```python
from build123d import *

# Parameters (mm, degrees)
EXTRUDE_6_DEPTH = 60


with BuildPart() as part:
    # Эскиз1 → Повернуть7 (revolve)
    with BuildSketch(Plane.XY, mode=Mode.PRIVATE) as revolve_7_sk:
        Polygon((120, 0), (0, 0), (0, -100), (90, -100), (90, -355), (20, -355), (20, -400), (40, -400), (115.131397208, -379.868602792), (120, -375), align=None)
    revolve(revolve_7_sk.sketch.rotate(Axis((0, 0, 0), (1, 0, 0)), 270), axis=Axis((0, 0, 0), (1, 0, 0)))

    # Эскиз3 → Бобышка-Вытянуть6 (add)
    with BuildSketch(Plane.ZY.offset(-90)):
        with BuildLine():
            ThreePointArc((-48.745403909, -87.314864701), (-70.710678119, -70.710678119), (-87.314864701, -48.745403909))
            ThreePointArc((-87.314864701, -48.745403909), (-86.141576096, -54.996690721), (-88.975283359, -60.691012112))
            Line((-88.975283359, -60.691012112), (-257.169911814, -228.885640567))
            ThreePointArc((-257.169911814, -228.885640567), (-264.676174548, -231.805098536), (-271.900138456, -228.243980661))
            ThreePointArc((-271.900138456, -228.243980661), (-226.413585645, -273.42620254), (-173.542276552, -309.690294083))
            ThreePointArc((-173.542276552, -309.690294083), (-203.646432227, -265.561170399), (-186.637594429, -214.921865676))
            Line((-186.637594429, -214.921865676), (-60.691012112, -88.975283359))
            ThreePointArc((-60.691012112, -88.975283359), (-54.996690721, -86.141576096), (-48.745403909, -87.314864701))
        make_face()
        with BuildLine():
            ThreePointArc((-96.209138584, -27.272727273), (-100, 0), (-96.209138584, 27.272727273))
            ThreePointArc((-96.209138584, 27.272727273), (-99.799825551, 22.022759648), (-105.830052443, 20))
            Line((-105.830052443, 20), (-343.693177122, 20))
            ThreePointArc((-343.693177122, 20), (-351.065274929, 23.243360753), (-353.655298198, 30.869565217))
            ThreePointArc((-353.655298198, 30.869565217), (-353.440103732, -33.242940208), (-341.697027586, -96.271186441))
            ThreePointArc((-341.697027586, -96.271186441), (-331.779877601, -43.780331217), (-283.94541729, -20))
            Line((-283.94541729, -20), (-105.830052443, -20))
            ThreePointArc((-105.830052443, -20), (-99.799825551, -22.022759648), (-96.209138584, -27.272727273))
        make_face()
        with BuildLine():
            ThreePointArc((-87.314864701, 48.745403909), (-70.710678119, 70.710678119), (-48.745403909, 87.314864701))
            ThreePointArc((-48.745403909, 87.314864701), (-54.996690721, 86.141576096), (-60.691012112, 88.975283359))
            Line((-60.691012112, 88.975283359), (-228.885640567, 257.169911814))
            ThreePointArc((-228.885640567, 257.169911814), (-231.805098536, 264.676174548), (-228.243980661, 271.900138456))
            ThreePointArc((-228.243980661, 271.900138456), (-273.42620254, 226.413585645), (-309.690294083, 173.542276552))
            ThreePointArc((-309.690294083, 173.542276552), (-265.561170399, 203.646432227), (-214.921865676, 186.637594429))
            Line((-214.921865676, 186.637594429), (-88.975283359, 60.691012112))
            ThreePointArc((-88.975283359, 60.691012112), (-86.141576096, 54.996690721), (-87.314864701, 48.745403909))
        make_face()
        with BuildLine():
            ThreePointArc((27.272727273, 96.209138584), (22.022759648, 99.799825551), (20, 105.830052443))
            Line((20, 105.830052443), (20, 343.693177122))
            ThreePointArc((20, 343.693177122), (23.243360753, 351.065274929), (30.869565217, 353.655298198))
            ThreePointArc((30.869565217, 353.655298198), (-33.242940208, 353.440103732), (-96.271186441, 341.697027586))
            ThreePointArc((-96.271186441, 341.697027586), (-43.780331217, 331.779877601), (-20, 283.94541729))
            Line((-20, 283.94541729), (-20, 105.830052443))
            ThreePointArc((-20, 105.830052443), (-22.022759648, 99.799825551), (-27.272727273, 96.209138584))
            ThreePointArc((-27.272727273, 96.209138584), (0, 100), (27.272727273, 96.209138584))
        make_face()
        with BuildLine():
            ThreePointArc((60.691012112, 88.975283359), (54.996690721, 86.141576096), (48.745403909, 87.314864701))
            ThreePointArc((48.745403909, 87.314864701), (70.710678119, 70.710678119), (87.314864701, 48.745403909))
            ThreePointArc((87.314864701, 48.745403909), (86.141576096, 54.996690721), (88.975283359, 60.691012112))
            Line((88.975283359, 60.691012112), (257.169911814, 228.885640567))
            ThreePointArc((257.169911814, 228.885640567), (264.676174548, 231.805098536), (271.900138456, 228.243980661))
            ThreePointArc((271.900138456, 228.243980661), (226.413585645, 273.42620254), (173.542276552, 309.690294083))
            ThreePointArc((173.542276552, 309.690294083), (203.646432227, 265.561170399), (186.637594429, 214.921865676))
            Line((186.637594429, 214.921865676), (60.691012112, 88.975283359))
        make_face()
        with BuildLine():
            ThreePointArc((105.830052443, 20), (99.799825551, 22.022759648), (96.209138584, 27.272727273))
            ThreePointArc((96.209138584, 27.272727273), (99.047750753, 13.767464211), (100, 0))
            ThreePointArc((100, 0), (99.047750753, -13.767464211), (96.209138584, -27.272727273))
            ThreePointArc((96.209138584, -27.272727273), (99.799825551, -22.022759648), (105.830052443, -20))
            Line((105.830052443, -20), (343.693177122, -20))
            ThreePointArc((343.693177122, -20), (351.065274929, -23.243360753), (353.655298198, -30.869565217))
            ThreePointArc((353.655298198, -30.869565217), (354.663665224, -15.449419727), (355, 0))
            ThreePointArc((355, 0), (351.658530959, 48.592978952), (341.697027586, 96.271186441))
            ThreePointArc((341.697027586, 96.271186441), (331.779877601, 43.780331217), (283.94541729, 20))
            Line((283.94541729, 20), (105.830052443, 20))
        make_face()
        with BuildLine():
            ThreePointArc((88.975283359, -60.691012112), (86.141576096, -54.996690721), (87.314864701, -48.745403909))
            ThreePointArc((87.314864701, -48.745403909), (70.710678119, -70.710678119), (48.745403909, -87.314864701))
            ThreePointArc((48.745403909, -87.314864701), (54.996690721, -86.141576096), (60.691012112, -88.975283359))
            Line((60.691012112, -88.975283359), (228.885640567, -257.169911814))
            ThreePointArc((228.885640567, -257.169911814), (231.805098536, -264.676174548), (228.243980661, -271.900138456))
            ThreePointArc((228.243980661, -271.900138456), (273.42620254, -226.413585645), (309.690294083, -173.542276552))
            ThreePointArc((309.690294083, -173.542276552), (265.561170399, -203.646432227), (214.921865676, -186.637594429))
            Line((214.921865676, -186.637594429), (88.975283359, -60.691012112))
        make_face()
        with BuildLine():
            ThreePointArc((20, -105.830052443), (22.022759648, -99.799825551), (27.272727273, -96.209138584))
            ThreePointArc((27.272727273, -96.209138584), (0, -100), (-27.272727273, -96.209138584))
            ThreePointArc((-27.272727273, -96.209138584), (-22.022759648, -99.799825551), (-20, -105.830052443))
            Line((-20, -105.830052443), (-20, -343.693177122))
            ThreePointArc((-20, -343.693177122), (-23.243360753, -351.065274929), (-30.869565217, -353.655298198))
            ThreePointArc((-30.869565217, -353.655298198), (33.242940208, -353.440103732), (96.271186441, -341.697027586))
            ThreePointArc((96.271186441, -341.697027586), (43.780331217, -331.779877601), (20, -283.94541729))
            Line((20, -283.94541729), (20, -105.830052443))
        make_face()
    extrude(amount=EXTRUDE_6_DEPTH)


solid = part.part
```
Work out the finished part from the listing and answer in its coordinate system (mm). Round coordinates to 2 decimals unless told otherwise and drop trailing zeros. Loops run counter-clockwise (first coordinate to the right, second up) from the corner with the lowest first, then second, coordinate; pieces in that order, holes last.
(1) Each of these flat-tipped pins is pushed along its axis until it touches: P1, Ø4, axis at x = 47.5, z = 98.5, coming from the +Y side; P2, Ø18, axis at x = 46.5, z = 215, coming from the -Y side; P3, Ø10, axis at x = 90, y = -226.5, coming from the -Z side. Where does it stop, or does it pass through?
Computed values:
P1: stops at y = 386.36
P2: stops at y = -341.53
P3: stops at z = -317.22
(2) The mould has two halves that part along Z. Classify faces 1 (the conical face through (119.764, 366.313, -81.344)), 2 (the flat face through (120, -5, -5)), 3 (the flat face through (30, 169, -170)): pulls with the +Z half, pulls with the -Z half, needs draft (parallel to the pull), parting line crosses it, or undercut.
Computed values:
face 1: parting line crosses it
face 2: needs draft
face 3: undercut
(3) The part is cut by section C-C, the plane x = 10.5. Give the vertices of the cut face in (y, z), and give its area (3 significant figures).
Computed values:
outline: circle Ø200 at (0, 0)
area: 31,400 mm2
(4) Find the intervals of material crossed by L1, parallel to Y at x = 71, z = 110; L2, parallel to Y at x = 36.5, z = 117; L3, parallel to Z at x = 28.5, y = -17.5, in increasing order.
Computed values:
L1: y = -375.93 to -337.53, -138.28 to -81.72, -20 to 20, 81.72 to 138.28, 337.53 to 375.93
L2: y = -382.51 to -335.17, -145.28 to -88.72, -20 to 20, 88.72 to 145.28, 335.17 to 382.51
L3: z = -399.62 to -354.57, -98.46 to 98.46, 354.57 to 399.62
(5) The part is cut by section D-D, the plane x = 78.5. Give the number of separate pieces and of enclosed holes in the cut face, and give its area (3 significant figures).
Computed values:
separate pieces: 1
enclosed holes: 8
area: 204,000 mm2
(6) The part is cut by section A-A, the plane y = 0. Give the vertices of the cut face in (x, z), and give its area (3 significant figures).
Computed values:
outline: (0, -100) - (30, -100) - (30, -355) - (20, -355) - (20, -400) - (40, -400) - (115.13, -379.87) - (120, -375) - (120, 375) - (115.13, 379.87) - (40, 400) - (20, 400) - (20, 355) - (30, 355) - (30, 100) - (0, 100) - close
area: 77,200 mm2
